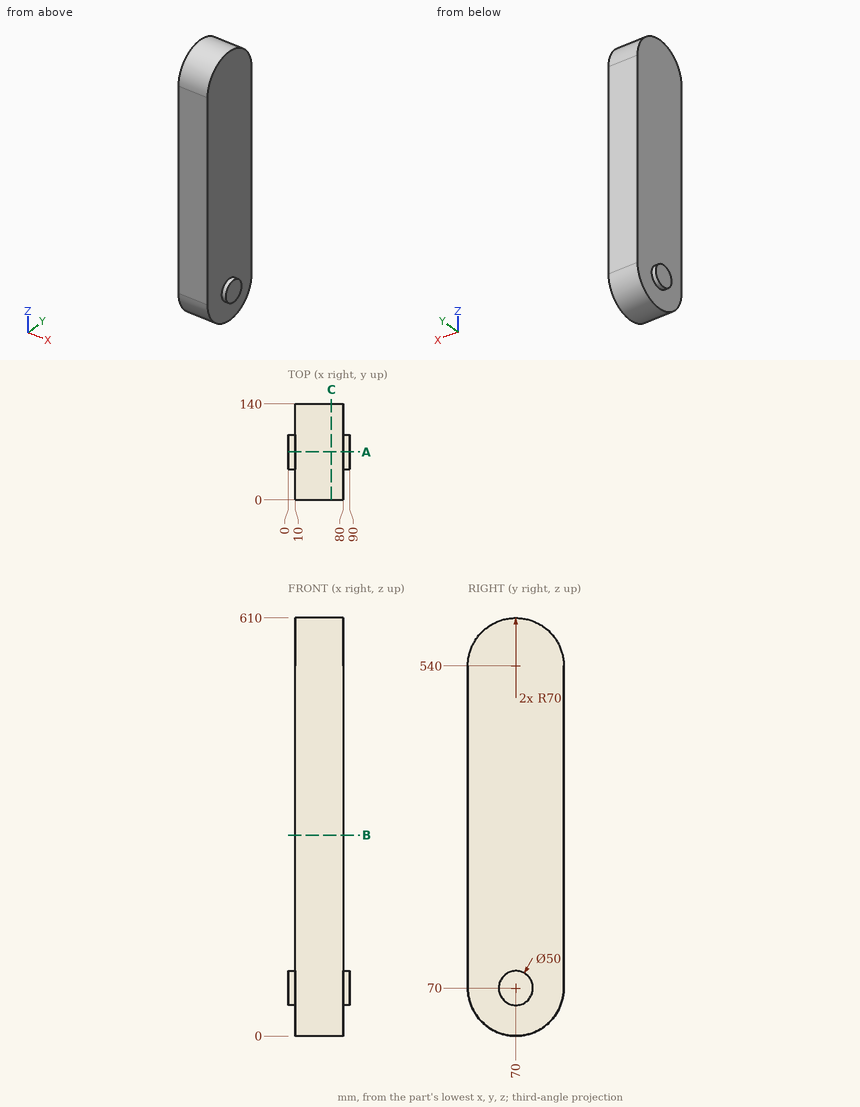
Verification items for this drawing (mm, ordinates from the low corner). Round coordinates to 2 decimals unless told otherwise and drop trailing zeros. Loops run counter-clockwise (first coordinate to the right, second up) from the corner with the lowest first, then second, coordinate; pieces in that order, holes last. Notation, with made-up numbers: (57.5, 49) - (77.5, 49) arc R9 ccw to (77.5, 63) - close; hole circle Ø11 at (-16.75, 63). An arc over 180 degrees is marked (long way). Write item = value, one per line.
Q1. Sectioned sample at A-A on y = 70. Record the boundary of the cut face in (x, z).
Here are the results:
outline = (0, 45) - (10, 45) - (10, 0) - (80, 0) - (80, 45) - (90, 45) - (90, 95) - (80, 95) - (80, 610) - (10, 610) - (10, 95) - (0, 95) - close
Q2. Sectioned sample at C-C on x = 63. Record the boundary of the cut face in (y, z), plus the area to 3 significant figures.
Here are the results:
outline = (0, 70) arc R70 ccw to (140, 70) - (140, 540) arc R70 ccw to (0, 540) - close
area = 81,200 mm^2
Q3. Depth check by flat-ended pin: pin 1 (10 mm diameter, centred on x = 75.5, y = 67.5, fed in from +Z); pin 2 (1 mm diameter, centred on y = 69.5, z = 188.5, fed in from +X); pin 3 (4 mm diameter, centred on y = 124, z = 275.5, fed in from -X). Enter the tip coordinate at first touch or a pass-through.
Here are the results:
pin_1 = 610
pin_2 = 80
pin_3 = 10
Q4. Material ranges on L1, parallel to X at y = 7, z = 440; L2, parallel to Y at x = 6, z = 59; L3, parallel to Z at x = 36.5, y = 111.5, recorded low to high.
Here are the results:
L1 = 10 to 80
L2 = 47.55 to 92.45
L3 = 13.63 to 596.37
Q5. Sectioned sample at B-B on z = 293. Record the boundary of the cut face in (x, y).
Here are the results:
outline = (10, 0) - (80, 0) - (80, 140) - (10, 140) - close
